Part model, mm, in its own coordinate system. A direction names the side the tool comes from. Round coordinates to 2 decimals unless told otherwise and drop trailing zeros. Loops run counter-clockwise (first coordinate to the right, second up) from the corner with the lowest first, then second, coordinate; pieces in that order, holes last. Notation, with made-up numbers: (-36, 8) -> (-22, 8) arc R8 cw to (-22, 20) -> close; hole circle Ø1 at (80, -15). An arc over 180 degrees is marked (long way). Use a Markdown table: item, result. Add a question column.
Item 1: Two-plate mould, pull along X, no slides. Class faces 1 (the face through (0.47, 37.94, 3.45)), 2 (the face through (4, 17, 0)), 3 (the face through (2.636, 21.285, 3.451)): pulls with the +X half, pulls with the -X half, needs draft (parallel to the pull), parting line crosses it, or undercut.
Item 2: Probe line 1 (Y direction, x = 8, z = 4.5); line 2 (X direction, y = 4, z = 3.75); line 3 (X direction, y = 12.5, z = 2.25). List the from-to ranges inside material, lowest first. Write a range as [from, to].
Item 3: Cut at C-C, the plane y = 2.5. List the corners of the cut face in (x, z), plus the area to 3 significant figures.
Item 4: Flat gauge pins, fed straight in: pin 1 (3 mm diameter, centred on y = 16.5, z = 5, fed in from +X); pin 2 (0.6 mm diameter, centred on y = 24, z = 3.5, fed in from +X). Where does each tip first touch, or does it go through?
Item 5: Cut at A-A, the plane z = 3.75. List the corners of the cut face in (x, y).
Item 6: Cut at D-D, the plane x = 9.25. List the corners of the cut face in (y, z).
Item 7: Which spindle directions (+Z, -Z, +X, -X, +Y, -Y) get a long thin tool onto all of the face, cutting with end or side? Do faces 4 (the face through (6.947, 24, 3)), 5 (the face through (10.52, 35.77, 3.55)), 6 (the face through (2.277, -9.089, 3.451)), 7 (the face through (11, 34.571, 3)). Say none if no direction does.
Item 8: Cut at B-B, the plane y = 19.5. List the corners of the cut face in (x, z), plus the area to 3 significant figures.
```python
from build123d import *

# Parameters (mm, degrees)
PAD_DEPTH   = 7
FILLET_R    = 0.5
FILLET001_R = 1
FILLET002_R = 1


with BuildPart() as part:
    # Sketch → Pad (new body)
    with BuildSketch(Plane.XY):
        with BuildLine():
            Line((1.140353, 38.211909), (6.608476, 38.211909))
            Line((12.389766, 38.211909), (6.608476, 38.211909))
            Line((12.389766, 34.571056), (12.389766, 38.211909))
            Line((10.843417, 34.571056), (12.389766, 34.571056))
            Line((10.781564, 36.055546), (10.843417, 34.571056))
            Line((3.792074, 36.055546), (10.781564, 36.055546))
            Line((3.792074, 23.437357), (3.792074, 36.055546))
            Line((3.792074, 23.437357), (5.64769, 23.437357))
            Line((5.64769, 23.437357), (5.64769, 24.674435))
            Line((5.64769, 24.674435), (6.946622, 24.674435))
            Line((6.946622, 24.674435), (6.946622, 23.394299))
            Line((6.946622, 23.394299), (7.230929, 23.394299))
            Line((7.230929, 23.394299), (5.878444, 13.2727))
            Line((4.444027, -8.845778), (5.878444, 13.2727))
            ThreePointArc((3.074544, -10.551747), (4.049152, -9.931456), (4.444027, -8.845778))
            ThreePointArc((2.99206, -7.068146), (2.588113, -8.820488), (3.074544, -10.551747))
            Line((3.393693, 20.659941), (2.99206, -7.068146))
            ThreePointArc((3.393693, 20.659941), (2.620383, 21.285237), (1.880762, 20.620434))
            Line((1.880762, 20.620434), (1.952176, -7.313535))
            ThreePointArc((1.895787, -10.802761), (2.277294, -9.063858), (1.952176, -7.313535))
            ThreePointArc((0.177781, -8.839589), (0.658741, -10.152007), (1.895787, -10.802761))
            Line((0.178586, 37.250143), (0.177781, -8.839589))
            ThreePointArc((1.140353, 38.211909), (0.460281, 37.930214), (0.178586, 37.250143))
        make_face()
    extrude(amount=PAD_DEPTH)

    # Fillet
    fillet_edges = [part.edges().sort_by_distance(p)[0] for p in [
        (12.389766, 34.571056, 3.5),
    ]]
    fillet(fillet_edges, radius=FILLET_R)

    # Fillet001
    fillet001_edges = [part.edges().sort_by_distance(p)[0] for p in [
        (12.389766, 38.211909, 3.5),
    ]]
    fillet(fillet001_edges, radius=FILLET001_R)

    # Fillet002
    fillet002_edges = [part.edges().sort_by_distance(p)[0] for p in [
        (10.781564, 36.055546, 3.5),
    ]]
    fillet(fillet002_edges, radius=FILLET002_R)


solid = part.part
```
A:
| question | item | result |
|---|---|---|
| 1 | face 1 | pulls with the -X half |
| 1 | face 2 | needs draft |
| 1 | face 3 | undercut |
| 2 | line 1 | y = [36.06, 38.21] |
| 2 | line 2 | x = [0.18, 1.92], [3.15, 5.28] |
| 2 | line 3 | x = [0.18, 1.9], [3.28, 5.83] |
| 3 | outline | (0.18, 0) -> (1.93, 0) -> (1.93, 7) -> (0.18, 7) -> close; (3.13, 0) -> (5.18, 0) -> (5.18, 7) -> (3.13, 7) -> close |
| 3 | area | 26.6 mm^2 |
| 4 | pin 1 | stops at x = 6.51 |
| 4 | pin 2 | stops at x = 6.95 |
| 5 | outline | (0.18, -8.84) arc R1.94 ccw to (1.9, -10.8) arc R4.48 ccw to (1.95, -7.31) -> (1.88, 20.62) arc R0.77 cw to (3.39, 20.66) -> (2.99, -7.07) arc R3.63 ccw to (3.07, -10.55) arc R1.8 ccw to (4.44, -8.85) -> (5.88, 13.27) -> (7.23, 23.39) -> (6.95, 23.39) -> (6.95, 24.67) -> (5.65, 24.67) -> (5.65, 23.44) -> (3.79, 23.44) -> (3.79, 36.06) -> (9.82, 36.06) arc R1 cw to (10.82, 35.1) -> (10.84, 34.57) -> (11.89, 34.57) arc R0.5 ccw to (12.39, 35.07) -> (12.39, 37.21) arc R1 ccw to (11.39, 38.21) -> (1.14, 38.21) arc R0.96 ccw to (0.18, 37.25) -> close |
| 6 | outline | (36.06, 0) -> (38.21, 0) -> (38.21, 7) -> (36.06, 7) -> close |
| 7 | face 4 | +Z, -Z, +X |
| 7 | face 5 | +Z, -Z, -Y |
| 7 | face 6 | +Z, -Z |
| 7 | face 7 | +Z, -Z, +X, -Y |
| 8 | outline | (0.18, 0) -> (1.88, 0) -> (1.88, 7) -> (0.18, 7) -> close; (3.38, 0) -> (6.71, 0) -> (6.71, 7) -> (3.38, 7) -> close |
| 8 | area | 35.3 mm^2 |
